Build history of the part. All positions in model axes, mm. A direction names the side the tool comes from. Round coordinates to 2 decimals unless told otherwise and drop trailing zeros. Write each loop counter-clockwise with the first axis right and the second up, starting at its lowest first coordinate (ties: lowest second). Pieces come first, ordered by that corner, then holes. Notation, with made-up numbers: M -3,-12.75 L 24,-12.75 A23 cw 24,12.25 Z; hole C 70.5,80 d8. An arc over 180 degrees is marked long. Write item = value, one per line. Start each with the question number.
Q1. Band-saw the part on C-C on z = -5. Write the cut outline in (x, y).
Q2. Band-saw the part on B-B on y = -6.5. Write the cut outline in (x, z).
Q3. Drop flat-ended pins along their axis: P1, Ø7, axis at x = -5, z = -24.75, coming from the -Y side; P2, Ø4.5, axis at x = -0.5, z = 24, coming from the +Y side; P3, Ø10, axis at x = 3.5, z = -23.5, coming from the -Y side. Give the stop position or say it passes through.
Q4. Band-saw the part on D-D on x = 5. Write the cut outline in (y, z).
Q5. Tool access for faces 1 (the cylindrical face through (9.4, -12.72, -19.43)), 2 (the cylindrical face through (9.4, 6.92, -19.43)), 3 (the cylindrical face through (-0.143, 16.412, -6.753)): list every direction of +Z, -Z, +X, -X, +Y, -Y with a clear straight run to the whole face (end or side of a thin tool).
Q6. Probe L1, parallel to X at y = 0.5, z = -24.75; L2, parallel to X at y = 1, z = 24; L3, parallel to Y at x = 3, z = 15.5. List the from-to ranges inside material, lowest first.
Q7. Band-saw the part on A-A on z = 24.75. Write the cut outline in (x, y), plus the area to 3 significant figures.
```python
from build123d import *

# Parameters (mm, degrees)
BOSS_EXTRUDE1_DEPTH      = 13.7
BOSS_EXTRUDE1_DEPTH_BACK = 27.8
SKETCH1_W                = 20
SKETCH1_H                = 40
SKETCH4_W                = 20
SKETCH4_H                = 54.5
BOSS_EXTRUDE2_DEPTH      = 2
SKETCH5_R                = 3
CUT_EXTRUDE1_DEPTH       = 42.600510814
SKETCH6_R                = 3.25
BOSS_EXTRUDE3_DEPTH      = 5.5
SKETCH7_W                = 6.666666666
SKETCH7_H                = 2
BOSS_EXTRUDE4_DEPTH      = 7.25
BOSS_EXTRUDE4_TAPER      = 2
FILLET1_R                = 2


with BuildPart() as part:
    # Sketch1 → Boss-Extrude1 (new, two sides: drawn at the far end of the back side and taken through both)
    with BuildSketch(Plane(origin=(0, 0, 0), x_dir=(1, 0, 0), z_dir=(0, 1, 0)).offset(-BOSS_EXTRUDE1_DEPTH_BACK)):
        Rectangle(SKETCH1_W, SKETCH1_H)
    extrude(amount=BOSS_EXTRUDE1_DEPTH + BOSS_EXTRUDE1_DEPTH_BACK)

    # Sketch4 → Boss-Extrude2 (add)
    with BuildSketch(Plane(origin=(0, 0, 0), x_dir=(1, 0, 0), z_dir=(0, 1, 0))):
        Rectangle(SKETCH4_W, SKETCH4_H)
    extrude(amount=BOSS_EXTRUDE2_DEPTH)

    # Sketch5 → Cut-Extrude1 (cut, through all)
    with BuildSketch(Plane(origin=(0, 2, 0), x_dir=(1, 0, 0), z_dir=(0, 1, 0))):
        with Locations((-5, 24.75)):
            Circle(SKETCH5_R)
        with Locations((5, 24.75)):
            Circle(SKETCH5_R)
        with Locations((-5, -24.75)):
            Circle(SKETCH5_R)
        with Locations((5, -24.75)):
            Circle(SKETCH5_R)
    extrude(amount=-CUT_EXTRUDE1_DEPTH, mode=Mode.SUBTRACT)

    # Sketch6 → Boss-Extrude3 (add)
    with BuildSketch(Plane(origin=(0, 13.7, 0), x_dir=(1, 0, 0), z_dir=(0, 1, 0))):
        with Locations(Location((0, 10, 0), (0, 0, 90))):
            Circle(SKETCH6_R)
    extrude(amount=BOSS_EXTRUDE3_DEPTH)

    # Sketch7 → Boss-Extrude4 (add)
    with BuildSketch(Plane(origin=(0, 0, -20), x_dir=(-1, 0, 0), z_dir=(0, 0, -1))):
        with Locations((0, -24.8)):
            Rectangle(SKETCH7_W, SKETCH7_H)
    extrude(amount=BOSS_EXTRUDE4_DEPTH, taper=BOSS_EXTRUDE4_TAPER)

    # Fillet1
    fillet1_edges = [part.edges().sort_by_distance(p)[0] for p in [
        (10, -27.8, 0),
        (0, -27.8, 20),
        (-10, -27.8, 0),
        (0, -27.8, -20),
        (-10, 13.7, 0),
        (0, 13.7, 20),
        (-10, -13.9, 20),
        (10, -13.9, 20),
        (-10, -13.9, -20),
        (10, -13.9, -20),
        (10, 13.7, 0),
        (10, 7.85, 20),
        (-10, 7.85, 20),
        (-10, 7.85, -20),
        (10, 7.85, -20),
        (0, 13.7, -20),
    ]]
    fillet(fillet1_edges, radius=FILLET1_R - 0.0001)  # a hair under: the kernel refuses the full size


solid = part.part
```
Conclusion:
q1.outline = M -10,-25.8 A2 ccw -8,-27.8 L 8,-27.8 A2 ccw 10,-25.8 L 10,11.7 A2 ccw 8,13.7 L -8,13.7 A2 ccw -10,11.7 Z
q2.outline = M -10,-18 A2 ccw -8,-20 L 8,-20 A2 ccw 10,-18 L 10,18 A2 ccw 8,20 L -8,20 A2 ccw -10,18 Z
q3.P1 = -25.74
q3.P2 = 2
q3.P3 = -27.74
q4.outline = M -27.8,-18 A2 ccw -25.8,-20 L 0,-20 L 0,-21.75 L 2,-21.75 L 2,-20 L 11.7,-20 A2 ccw 13.7,-18 L 13.7,18 A2 ccw 11.7,20 L 2,20 L 2,21.75 L 0,21.75 L 0,20 L -25.8,20 A2 ccw -27.8,18 Z
q5.face_1 = -Z, +X, -Y
q5.face_2 = -Z, +X, +Y
q5.face_3 = +Y
q6.L1 = -10 to -8, -2 to 2, 8 to 10
q6.L2 = -10 to -7.9, -2.1 to 2.1, 7.9 to 10
q6.L3 = -27.8 to 13.7
q7.outline = M -10,0 L -8,0 L -8,2 L -10,2 Z; M -2,0 L 2,0 L 2,2 L -2,2 Z; M 8,0 L 10,0 L 10,2 L 8,2 Z
q7.area = 16.0 mm^2
